Build history of the part. All positions in model axes, mm. A direction names the side the tool comes from. Give positions to 0.01 mm unless a question says otherwise; leave off trailing zeros. Order: outer loops, then holes, each group sorted by start corner. A loop starts at its lowest first (then second) coordinate and runs counter-clockwise, first axis right, second up. Notation, with made-up numbers: (-7, 72.5) - (48, 72.5) arc R10 ccw to (48, 82.5) - close; hole circle Ø9 at (-6, 27). An arc over 180 degrees is marked (long way). Use a Markdown table: item, result. Add a question column.
(1) Slice it at A-A (y = 0.9). Write the cut outline in (x, z).
(2) Slice it at B-B (x = 4). Write the cut outline in (y, z), then the cut area to 3 significant figures.
(3) Mould opens along Z. For faces 1 (the face through (15.336, 1.479, 0.575)), 2 (the face through (60.096, 1.479, -14.513)), 3 (the face through (-59.64, 1.48, 0.31)) say: +Z half, -Z half, draft (parallel to the pull), parting line (faces both ways), or undercut.
(4) Which spindle directions (+Z, -Z, +X, -X, +Y, -Y) get a long thin tool onto all of the face, cutting with end or side? Do faces 4 (the face through (-23.7, 1.5, 17.1)), 5 (the face through (11.25, 1, 0)). Say none if no direction does.
(5) Wall check: line 1 (X direction, y = 0.8, z = -4); line 2 (X direction, y = 1.7, z = -3.5); line 3 (Z direction, x = 120, y = 1.1). Give the ranges that are in metal, low to high.
(6) Flat gauge pins, fed straight in: pin 1 (5 mm diameter, centred on x = -13.95, z = 0, fed in from -Y); pin 2 (1.5 mm diameter, centred on y = 2, z = 1.5, fed in from +X); pin 3 (1.5 mm diameter, centred on y = 2.5, z = 6, fed in from +X); pin 4 (0.9 mm diameter, centred on x = -5, y = 2, fed in from +Z). Where does each tip first touch, or does it go through?
from build123d import *

# Parameters (mm, degrees)
SKETCH1_R           = 1.5
SKETCH1_R_2         = 3
SKETCH1_W           = 22.5
SKETCH1_H           = 12.2
BOSS_EXTRUDE1_DEPTH = 3


with BuildPart() as part:
    # Sketch1 → Boss-Extrude1 (new body)
    with BuildSketch(Plane(origin=(0, 0, 0), x_dir=(1, 0, 0), z_dir=(0, 1, 0))):
        with BuildLine():
            Line((1.846751087, 19.91455524), (120, 8.957763171))
            ThreePointArc((120, 8.957763171), (128.957763171, 0), (120, -8.957763171))
            Line((120, -8.957763171), (1.846751087, -19.91455524))
            Line((1.846751087, -19.91455524), (-2.565887989, -19.834722555))
            Line((-2.565887989, -19.834722555), (-45.343490518, -14.300864634))
            ThreePointArc((-45.343490518, -14.300864634), (-59.644355152, 0), (-45.343490518, 14.300864634))
            Line((-45.343490518, 14.300864634), (-2.565887989, 19.834722555))
            Line((-2.565887989, 19.834722555), (1.846751087, 19.91455524))
        make_face()
        with Locations((13.95, 0)):
            Circle(SKETCH1_R, mode=Mode.SUBTRACT)
        with Locations((-13.95, 0)):
            Circle(SKETCH1_R, mode=Mode.SUBTRACT)
        with Locations((120, 0)):
            Circle(SKETCH1_R_2, mode=Mode.SUBTRACT)
        Rectangle(SKETCH1_W, SKETCH1_H, mode=Mode.SUBTRACT)
        Polygon((96.529167285, 4.104267173), (67.660347399, 6.781380665), (67.660347399, -6.781380665), (96.529167285, -4.104267173), align=None, mode=Mode.SUBTRACT)
        Polygon((59.65913304, 7.523363157), (26.779600723, 10.572404992), (26.779600723, -10.572404992), (59.65913304, -7.523363157), align=None, mode=Mode.SUBTRACT)
    extrude(amount=BOSS_EXTRUDE1_DEPTH)


solid = part.part
Solution:
| question | item | result |
|---|---|---|
| 1 | outline | (-45.34, -14.3) - (-2.57, -19.83) - (1.85, -19.91) - (120, -8.96) arc R8.96 ccw to (120, 8.96) - (1.85, 19.91) - (-2.57, 19.83) - (-45.34, 14.3) arc R14.3 ccw to start; hole circle Ø3 at (-13.95, 0); hole (-11.25, -6.1) - (11.25, -6.1) - (11.25, 6.1) - (-11.25, 6.1) - close; hole circle Ø3 at (13.95, 0); hole (26.78, -10.57) - (59.66, -7.52) - (59.66, 7.52) - (26.78, 10.57) - close; hole (67.66, -6.78) - (96.53, -4.1) - (96.53, 4.1) - (67.66, 6.78) - close; hole circle Ø6 at (120, 0) |
| 2 | outline | (0, -19.71) - (3, -19.71) - (3, -6.1) - (0, -6.1) - close; (0, 6.1) - (3, 6.1) - (3, 19.71) - (0, 19.71) - close |
| 2 | area | 81.7 mm2 |
| 3 | face 1 | undercut |
| 3 | face 2 | -Z half |
| 3 | face 3 | parting line |
| 4 | face 4 | +Z, -X, +Y, -Y |
| 4 | face 5 | +Y, -Y |
| 5 | line 1 | -59.07 to -11.25, 11.25 to 26.78, 59.66 to 67.66, 96.53 to 128.02 |
| 5 | line 2 | -59.21 to -11.25, 11.25 to 26.78, 59.66 to 67.66, 96.53 to 128.25 |
| 5 | line 3 | -8.96 to -3, 3 to 8.96 |
| 6 | pin 1 | y = 0 |
| 6 | pin 2 | x = 128.93 |
| 6 | pin 3 | x = 127.26 |
| 6 | pin 4 | z = 19.58 |
